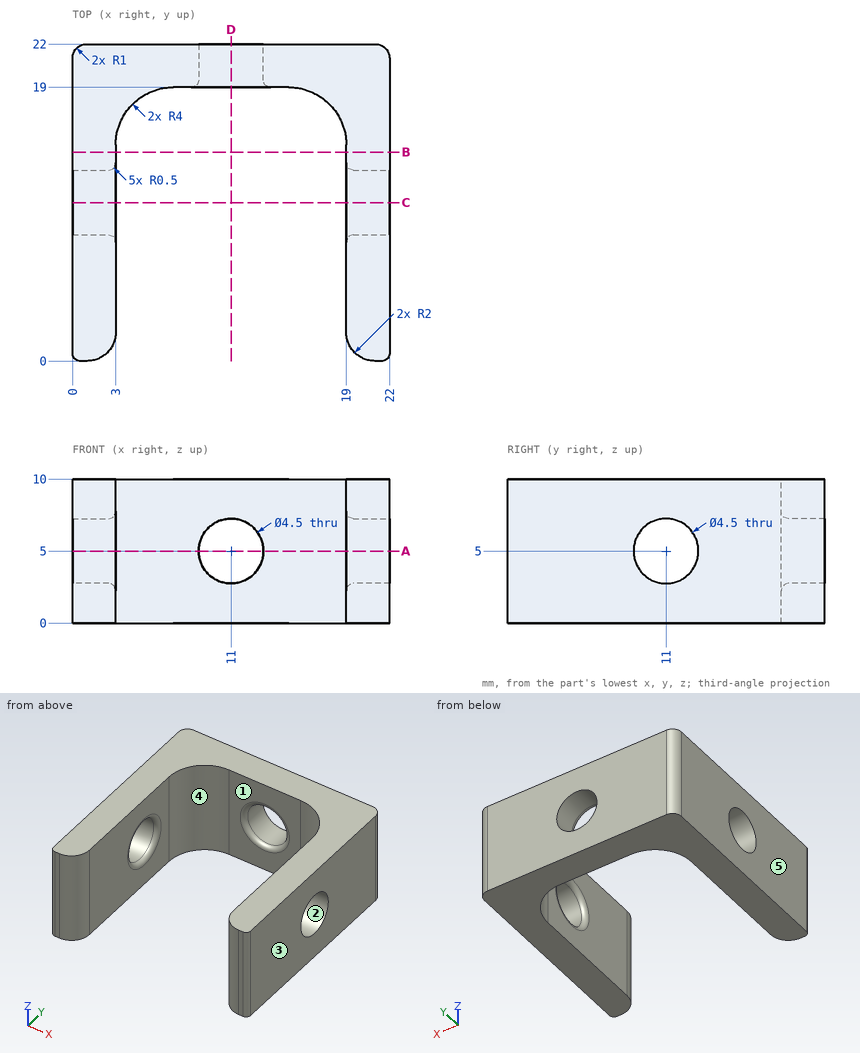
Drawing for the job (mm, zero at the part's lowest x, y, z). A direction names the side the tool comes from. Round coordinates to 2 decimals unless told otherwise and drop trailing zeros. Loops run counter-clockwise (first coordinate to the right, second up) from the corner with the lowest first, then second, coordinate; pieces in that order, holes last.
1. Mould opens along X. For the marked faces 3, 4 and 5 say: +X half, -X half, draft (parallel to the pull), parting line (faces both ways), or undercut.
Check values:
face 3: +X half
face 4: undercut
face 5: -X half
2. Band-saw the part on D-D, the plane x = 11. List the corners of the cut face in (y, z).
Check values:
outline: (19, 0) - (22, 0) - (22, 2.75) - (19.5, 2.75) arc R0.5 ccw to (19, 2.25) - close; (19, 7.75) arc R0.5 ccw to (19.5, 7.25) - (22, 7.25) - (22, 10) - (19, 10) - close
3. Drop flat-ended pins along their axis: P1, Ø5, axis at x = 4, z = 1.5, coming from the -Y side; P2, Ø2, axis at x = 9.5, z = 7.5, coming from the -Y side; P3, Ø1, axis at y = 10, z = 4, coming from the -X side; P4, Ø3, axis at x = 16, z = 3.5, coming from the -Y side. Give the stop position or say it passes through.
Check values:
P1: stops at y = 0.06
P2: stops at y = 19
P3: passes through
P4: stops at y = 18.12
4. Tool access for the marked faces 1 and 2: list every direction of +Z, -Z, +X, -X, +Y, -Y with a clear straight run to the whole face (end or side of a thin tool).
Check values:
face 1: +Z, -Z, -Y
face 2: +X, -X
5. Band-saw the part on B-B, the plane y = 14.5. List the corners of the cut face in (x, z).
Check values:
outline: (0, 0) - (3, 0) - (3, 10) - (0, 10) - close; (19, 0) - (22, 0) - (22, 10) - (19, 10) - close
6. Wall check: probe 1 along Z at (x, y) = (11, 20.6); probe 2 along X at (y, z) = (14.25, 6.5); probe 3 along X at (y, z) = (20.4, 5). Give the ranges that are in metal, low to high.
Check values:
probe 1: z = 0 to 2.75, 7.25 to 10
probe 2: x = 0 to 3, 19 to 22
probe 3: x = 0 to 8.75, 13.25 to 22
7. Band-saw the part on A-A, the plane z = 5. Count the separate pieces of the cut face and the enclosed holes in it, and give its area (3 significant figures).
Check values:
separate pieces: 4
enclosed holes: 0
area: 144 mm2
8. Band-saw the part on C-C, the plane y = 11. List the corners of the cut face in (x, z), and give its area (3 significant figures).
Check values:
outline: (0, 0) - (3, 0) - (3, 2.25) arc R0.5 ccw to (2.5, 2.75) - (0, 2.75) - close; (0, 7.25) - (2.5, 7.25) arc R0.5 ccw to (3, 7.75) - (3, 10) - (0, 10) - close; (19, 0) - (22, 0) - (22, 2.75) - (19.5, 2.75) arc R0.5 ccw to (19, 2.25) - close; (19, 7.75) arc R0.5 ccw to (19.5, 7.25) - (22, 7.25) - (22, 10) - (19, 10) - close
area: 32.8 mm2
